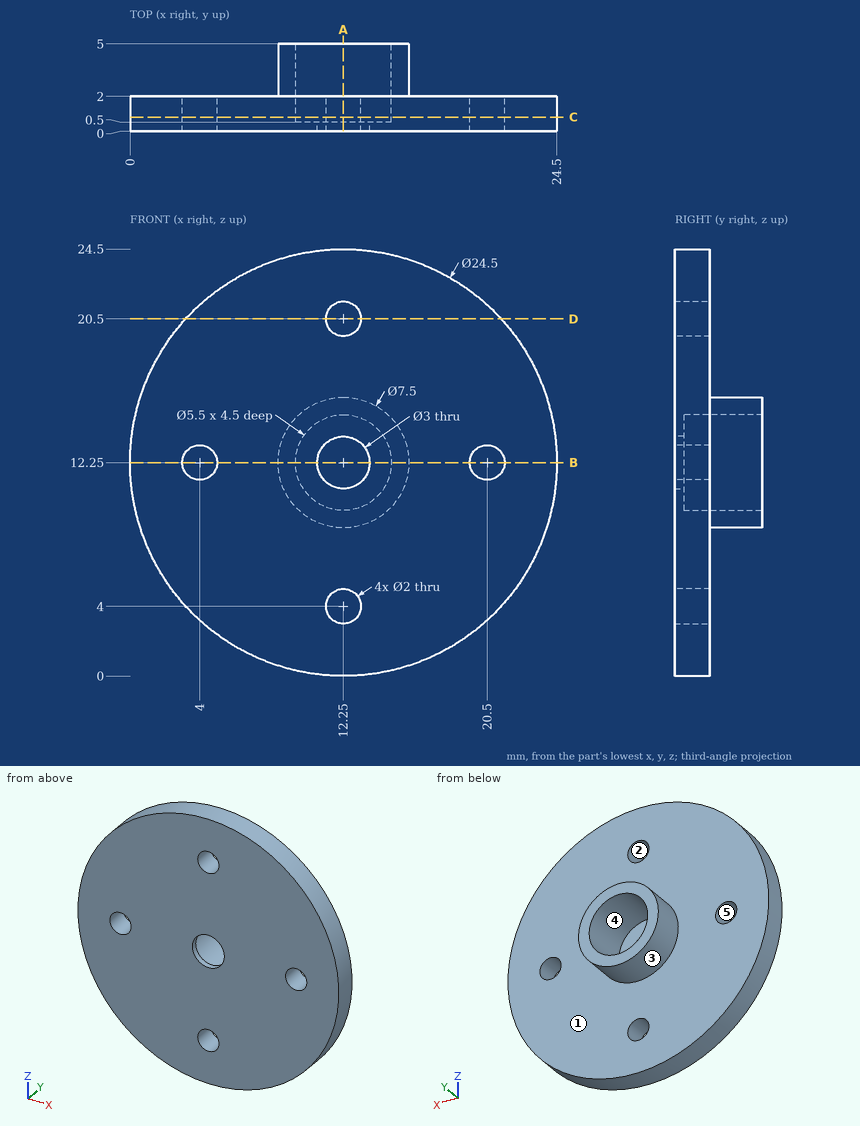
Can you work these out from the drawing? Everything is in mm from the part's minimum corner. A direction names the side the tool comes from. Give positions to 0.01 mm unless a question says otherwise; leave off trailing zeros. Loops run counter-clockwise (first coordinate to the right, second up) from the corner with the lowest first, then second, coordinate; pieces in that order, holes last. Notation, with made-up numbers: (-24, -29) - (30, -29) arc R5 cw to (30, -24) - close; hole circle Ø10 at (5.25, 89.5). An arc over 180 degrees is marked (long way). Use one line per item in the form item = value.
1. I want a section at A-A (x = 12.25). Please give me the cut outline in (y, z), and give its area (4 significant figures).
Response values:
outline = (0, 0) - (2, 0) - (2, 3) - (0, 3) - close; (0, 5) - (2, 5) - (2, 8.5) - (5, 8.5) - (5, 9.5) - (0.5, 9.5) - (0.5, 10.75) - (0, 10.75) - close; (0, 13.75) - (0.5, 13.75) - (0.5, 15) - (5, 15) - (5, 16) - (2, 16) - (2, 19.5) - (0, 19.5) - close; (0, 21.5) - (2, 21.5) - (2, 24.5) - (0, 24.5) - close
area = 37.25 mm²
2. I'm going to push flat-ended pins straight in: pin 1 Ø1.8 at (x, z) = (12.25, 4) entering from +Y; pin 2 Ø2.5 at (x, z) = (20.5, 12.25) entering from +Y; pin 3 Ø3 at (y, z) = (2.5, 14) entering from -X; pin 4 Ø2 at (x, y) = (9.5, 4.5) entering from -Z. Where does each tip first touch, or does it pass through?
Response values:
pin_1 = through
pin_2 = 2
pin_3 = 0
pin_4 = 8.93
3. I want a section at D-D (z = 20.5). Please give me the cut outline in (x, y), and give its area (3 significant figures).
Response values:
outline = (3.19, 0) - (11.25, 0) - (11.25, 2) - (3.19, 2) - close; (13.25, 0) - (21.31, 0) - (21.31, 2) - (13.25, 2) - close
area = 32.2 mm²
4. I want a section at B-B (z = 12.25). Please give me the cut outline in (x, y).
Response values:
outline = (0, 0) - (3, 0) - (3, 2) - (0, 2) - close; (5, 0) - (10.75, 0) - (10.75, 0.5) - (9.5, 0.5) - (9.5, 5) - (8.5, 5) - (8.5, 2) - (5, 2) - close; (13.75, 0) - (19.5, 0) - (19.5, 2) - (16, 2) - (16, 5) - (15, 5) - (15, 0.5) - (13.75, 0.5) - close; (21.5, 0) - (24.5, 0) - (24.5, 2) - (21.5, 2) - close
5. I need wall thicknesses on probe 1 along X at (y, z) = (0.3, 12.25); probe 2 along Z at (x, y) = (12.5, 1.5); probe 3 along Y at (x, z) = (17, 1.5). Which ranges of each line are inside material? Lowest first, please.
Response values:
probe_1 = 0 to 3, 5 to 10.75, 13.75 to 19.5, 21.5 to 24.5
probe_2 = 0 to 3.03, 4.97 to 9.51, 14.99 to 19.53, 21.47 to 24.5
probe_3 = 0 to 2
6. Thinking about a two-plate mould opening in Z: for the marked faces 1, 2 and 3, which applies, released by +Z, released by -Z, zero draft, split by the parting line, or undercut?
Response values:
face_1 = zero draft
face_2 = undercut
face_3 = split by the parting line
7. On a 3-axis mill with a long thin cutter (end or side, diameter ignored), from which of +Z, -Z, +X, -X, +Y, -Y can I reach the whole of each face in a straight line? I mean the marked faces 4 and 5. Say none if no direction works.
Response values:
face_4 = +Y
face_5 = +Y, -Y
8. I want a section at C-C (y = 0.8). Please give me the cut outline in (x, z), and give its area (3 significant figures).
Response values:
outline = circle Ø24.5 at (12.25, 12.25); hole circle Ø2 at (4, 12.25); hole circle Ø5.5 at (12.25, 12.25); hole circle Ø2 at (12.25, 4); hole circle Ø2 at (12.25, 20.5); hole circle Ø2 at (20.5, 12.25)
area = 435 mm²
